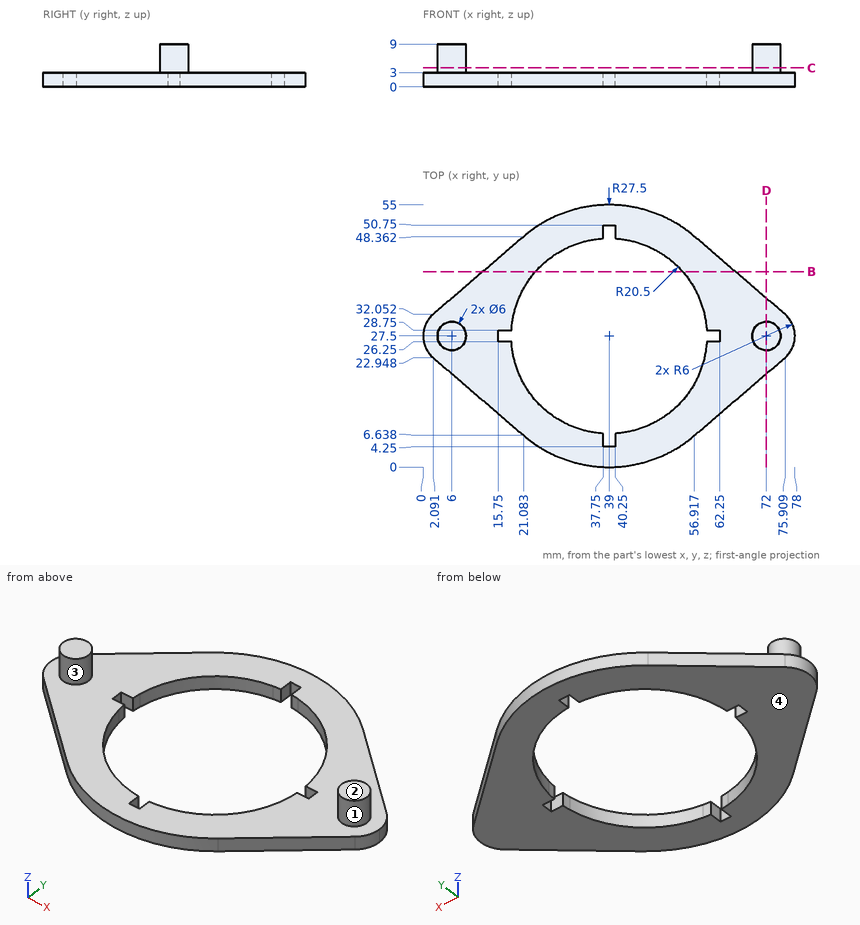
Study the drawing (mm; zero at the part's minimum x, y, z) and answer. A direction names the side the tool comes from. Coordinates: 2 decimals unless noted, no trailing zeros. Loops run counter-clockwise (first coordinate to the right, second up) from the corner with the lowest first, then second, coordinate; pieces in that order, holes last. Notation, with made-up numbers: M 55.25,43 L 109.25,43 A19 ccw 109.25,56 Z; hole C 71,65.5 d4. An arc over 180 degrees is marked long. Answer in a Markdown table with one row per item.
1) Find section D-D (x = 72). Determine the outline of the cut face in (y, z).
Answers below:
| item | result |
|---|---|
| outline | M 19.59,0 L 35.41,0 L 35.41,3 L 30.5,3 L 30.5,9 L 24.5,9 L 24.5,3 L 19.59,3 Z |
2) Given pin 1 (0.8 mm diameter, centred on y = 49, z = 2, fed in from -X) (1 decimal); pin 2 (3 mm diameter, centred on y = 5, z = 1, fed in from -X) (1 decimal); pin 3 (0.8 mm diameter, centred on y = 49.5, z = 1, fed in from +X), each flat-ended and moving along its own axis, determine where each tip first touches the part or whether it passes through.
Answers below:
| item | result |
|---|---|
| pin 1 | x = 21.4 |
| pin 2 | x = 21.2 |
| pin 3 | x = 56.02 |
3) Which of the six approach directions +Z, -Z, +X, -X, +Y, -Y give full straight-line access (tool end or side, diameter ignored) to the marked faces 3 and 4?
Answers below:
| item | result |
|---|---|
| face 3 | +Z |
| face 4 | -Z, +X, -X, +Y, -Y |
4) Find section B-B (y = 41). Determine the outline of the cut face in (x, z).
Answers below:
| item | result |
|---|---|
| outline | M 12.51,0 L 23.57,0 L 23.57,3 L 12.51,3 Z; M 54.43,0 L 65.49,0 L 65.49,3 L 54.43,3 Z |
5) Determine the mould class of the marked faces 1 and 2 for opening direction X: released by +X, released by -X, zero draft, split by the parting line, or undercut.
Answers below:
| item | result |
|---|---|
| face 1 | undercut |
| face 2 | zero draft |
6) Find section C-C (z = 4). Determine the outline of the cut face in (x, y).
Answers below:
| item | result |
|---|---|
| outline | C 6,27.5 d6; C 72,27.5 d6 |
7) Find the intervals of material crossed by probe 1 along X at (y, z) = (24.5, 2.25) (1 decimal); probe 2 along Z at (x, y) = (13, 23); probe 3 along X at (y, z) = (24, 2.25) (1 decimal), in increasing order.
Answers below:
| item | result |
|---|---|
| probe 1 | 0.8 to 18.7, 59.3 to 77.2 |
| probe 2 | 0 to 3 |
| probe 3 | 1.1 to 18.8, 59.2 to 76.9 |
